Can you work these out from the model? Positions are in its coordinate system, mm. A direction names the side the tool comes from. Give positions to 0.01 mm unless a question says otherwise; leave off trailing zeros. Order: outer loops, then holes, each group sorted by start corner. A loop starts at its lowest first (then second) coordinate and runs counter-clockwise, first axis right, second up. Notation, with made-up numbers: (39.5, 41) - (94.5, 41) arc R15 cw to (94.5, 62) - close; hole circle Ø10 at (46, 82.5). An arc over 180 degrees is marked (long way). Answer as a JSON object with one key per item and string values.
```python
from build123d import *

# Parameters (mm, degrees)
CHAMFER1_SIZE  = 0.47037037
CHAMFER1_SIZE2 = 0.81470538


with BuildPart() as part:
    # Sketch1 → Revolve1 (revolve)
    with BuildSketch(Plane.XY):
        Polygon((0, 0), (-9.5377, 0), (-9.5377, 4.60375), (-8.001, 4.60375), (-8.001, 7.14375), (-9.5377, 7.14375), (-9.5377, 9.652), (0, 9.652), align=None)
    revolve(axis=Axis((0, 0, 0), (0, 1, 0)))

    # Chamfer1
    chamfer1_edges = [part.edges().sort_by_distance(p)[0] for p in [
        (9.5377, 9.652, 0),
    ]]
    chamfer1_side = [part.faces().sort_by_distance(p)[0] for p in [
        (0, 9.652, 0),
    ]]
    chamfer(chamfer1_edges, length=CHAMFER1_SIZE, length2=CHAMFER1_SIZE2, reference=chamfer1_side[0])


solid = part.part
```
Q1. If we section it at B-B, the plane x = 0: Please give me the cut outline in (y, z), then the cut area to 3 significant figures.
Recorded:
{"outline": "(0, -9.54) - (4.6, -9.54) - (4.6, -8) - (7.14, -8) - (7.14, -9.54) - (8.84, -9.54) - (9.65, -9.07) - (9.65, 9.07) - (8.84, 9.54) - (7.14, 9.54) - (7.14, 8) - (4.6, 8) - (4.6, 9.54) - (0, 9.54) - close", "area": "176 mm^2"}
Q2. Which directions (+Z, -Z, +X, -X, +Y, -Y) give clear straight access to the entire face, cutting with the end or side of a thin tool? Please do faces 1 (the face through (-2, 7.144, 8)), 2 (the face through (2.07, 8, -9.31)).
Recorded:
{"face 1": "none", "face 2": "+Y, -Y"}
Q3. If we section it at A-A, the plane z = 0: Please give me the cut outline in (x, y).
Recorded:
{"outline": "(-9.54, 0) - (9.54, 0) - (9.54, 4.6) - (8, 4.6) - (8, 7.14) - (9.54, 7.14) - (9.54, 8.84) - (9.07, 9.65) - (-9.07, 9.65) - (-9.54, 8.84) - (-9.54, 7.14) - (-8, 7.14) - (-8, 4.6) - (-9.54, 4.6) - close"}
Q4. We'd pull the mould along Y, two halves only. Please class faces 3 (the face through (1.73, 5.89, -7.81)), 4 (the face through (0, 0, 0)), 5 (the face through (2, 4.604, 8)), 6 (the face through (0, 9.652, 0)): released by +Y, released by -Y, zero draft, split by the parting line, or undercut.
Recorded:
{"face 3": "undercut", "face 4": "released by -Y", "face 5": "undercut", "face 6": "released by +Y"}
Q5. I need wall thicknesses on L1, parallel to Y at x = 8.25, z = 1.5; L2, parallel to Z at x = 0, y = 7.75; L3, parallel to Y at x = 7, z = 6. Which ranges of each line are inside material? Lowest first, please.
Recorded:
{"L1": "y = 0 to 4.6, 7.14 to 9.65", "L2": "z = -9.54 to 9.54", "L3": "y = 0 to 4.6, 7.14 to 9.39"}
Q6. I'm going to push flat-ended pins straight in: pin 1 Ø1.5 at (x, y) = (-5, 6) entering from -Z; pin 2 Ø5 at (y, z) = (8, 3) entering from +X; pin 3 Ø3 at (x, y) = (-6, 5.5) entering from -Z. Where does each tip first touch, or does it pass through?
Recorded:
{"pin 1": "stops at z = -6.78", "pin 2": "stops at x = 9.52", "pin 3": "stops at z = -8.24"}
